```python
from build123d import *

# Parameters (mm, degrees)
BOSS_EXTRUDE1_DEPTH = 22.225
BOSS_EXTRUDE2_DEPTH = 3.175
SKETCH4_R           = 1.000000032
CUT_EXTRUDE2_DEPTH  = 67.374967797
SKETCH5_R           = 2.000000064
CUT_EXTRUDE3_DEPTH  = 69.585879378
SKETCH6_W           = 19.999999878
SKETCH6_H           = 40.899999988
CUT_EXTRUDE4_DEPTH  = 69.585879378
SKETCH7_W           = 1.500000048
SKETCH7_H           = 1.000000032
CUT_EXTRUDE5_DEPTH  = 6.604
CUT_EXTRUDE6_START  = 40.9
SKETCH7_2_W         = 1.500000048
SKETCH7_2_H         = 1.000000032
CUT_EXTRUDE6_DEPTH  = 6.604


with BuildPart() as part:
    # Sketch1 → Boss-Extrude1 (new, symmetric)
    with BuildSketch(Plane.XY):
        Polygon((0, 0), (0, 63.5), (3.175, 63.5), (3.175, 3.175), (16.51, 3.175), (16.51, 0), align=None)
    extrude(amount=BOSS_EXTRUDE1_DEPTH, both=True)

    # Sketch3 → Boss-Extrude2 (add)
    with BuildSketch(Plane.XY.offset(22.225)):
        Polygon((3.175, 63.5), (16.51, 3.175), (3.175, 3.175), align=None)
    boss_extrude2 = extrude(amount=-BOSS_EXTRUDE2_DEPTH)

    # Mirror1: Boss-Extrude2 across plane
    add(boss_extrude2.mirror(Plane.XY))

    # Sketch4 → Cut-Extrude2 (cut, through all)
    with BuildSketch(Plane(origin=(0, 3.175, 0), x_dir=(1, 0, 0), z_dir=(0, 1, 0))):
        with Locations(Location((8.679999912, 12.7, 0), (0, 0, 180))):
            Circle(SKETCH4_R)
        with Locations((8.679999912, -12.7)):
            Circle(SKETCH4_R)
    extrude(amount=-CUT_EXTRUDE2_DEPTH, mode=Mode.SUBTRACT)

    # Sketch5 → Cut-Extrude3 (cut, through all)
    with BuildSketch(Plane(origin=(3.175, 0, 0), x_dir=(0, 0, -1), z_dir=(1, 0, 0))):
        with Locations(Location((-4.953, 5.874999934, 0), (0, 0, 90))):
            Circle(SKETCH5_R)
        with Locations(Location((5.047000066, 5.874999934, 0), (0, 0, 90))):
            Circle(SKETCH5_R)
        with Locations(Location((-4.953, 54.475000016, 0), (0, 0, 90))):
            Circle(SKETCH5_R)
        with Locations(Location((5.047000066, 54.475000016, 0), (0, 0, 90))):
            Circle(SKETCH5_R)
    extrude(amount=-CUT_EXTRUDE3_DEPTH, mode=Mode.SUBTRACT)

    # Sketch6 → Cut-Extrude4 (cut, through all)
    with BuildSketch(Plane(origin=(3.175, 0, 0), x_dir=(0, 0, -1), z_dir=(1, 0, 0))):
        with Locations((0.047000033, 30.174999975)):
            Rectangle(SKETCH6_W, SKETCH6_H)
    extrude(amount=-CUT_EXTRUDE4_DEPTH, mode=Mode.SUBTRACT)

    # Sketch7 → Cut-Extrude5 (cut)
    with BuildSketch(Plane.XZ.offset(-50.624999969)):
        with Locations((2.424999976, 0)):
            Rectangle(SKETCH7_W, SKETCH7_H)
    extrude(amount=-CUT_EXTRUDE5_DEPTH, mode=Mode.SUBTRACT)

    # Sketch7<2> → Cut-Extrude6 (cut)
    with BuildSketch(Plane.XZ.offset(-50.624999969).offset(CUT_EXTRUDE6_START)):
        with Locations((2.424999976, 0)):
            Rectangle(SKETCH7_2_W, SKETCH7_2_H)
    extrude(amount=CUT_EXTRUDE6_DEPTH, mode=Mode.SUBTRACT)


solid = part.part
```
Source: CAD feature listing. Evaluate the final solid. Frame: model axes, mm. A direction names the side the tool comes from. Round coordinates to 2 decimals unless told otherwise and drop trailing zeros. Loops run counter-clockwise (first coordinate to the right, second up) from the corner with the lowest first, then second, coordinate; pieces in that order, holes last.
(1) Material intervals for probe 1 along Z at (x, y) = (8.68, 1.1) (3 decimals); probe 2 along Y at (x, z) = (2.75, 6.5) (3 decimals); probe 3 along Z at (x, y) = (2.75, 33) (3 decimals), sorted ascending.
From the geometry:
probe 1: z = -22.225 to -13.7, -11.7 to 11.7, 13.7 to 22.225
probe 2: y = 0 to 4.607, 7.143 to 9.725, 50.625 to 53.207, 55.743 to 63.5
probe 3: z = -22.225 to -10.047, 9.953 to 22.225
(2) Access query for faces 1 (the flat face through (1, 9.725, 0)), 2 (the flat face through (2, 54, 0.5)), 3 (the flat face through (7, 20, 19.05)). Directions: +Z, -Z, +X, -X, +Y, -Y. A direction counts if a zero-diameter tool reaches every point of the face in a straight line with its end or side. Return the directions, or none.
From the geometry:
face 1: +X, -X
face 2: +X
face 3: +X, +Y
(3) Section query C-C (x = 8.68). Output: boundary loops of the cut face in (y, z) (3 decimals), and give its area (3 significant figures).
From the geometry:
outline: (0, -22.225) - (38.596, -22.225) - (38.596, -19.05) - (3.175, -19.05) - (3.175, -13.7) - (0, -13.7) - close; (0, -11.7) - (3.175, -11.7) - (3.175, 11.7) - (0, 11.7) - close; (0, 13.7) - (3.175, 13.7) - (3.175, 19.05) - (38.596, 19.05) - (38.596, 22.225) - (0, 22.225) - close
area: 353 mm2
(4) Section query D-D (y = 54). Output: boundary loops of the cut face in (x, z) (3 decimals), and give its area (3 significant figures).
From the geometry:
outline: (0, -22.225) - (5.275, -22.225) - (5.275, -19.05) - (3.175, -19.05) - (3.175, -6.99) - (0, -6.99) - close; (0, -3.104) - (3.175, -3.104) - (3.175, -0.5) - (1.675, -0.5) - (1.675, 0.5) - (3.175, 0.5) - (3.175, 3.01) - (0, 3.01) - close; (0, 6.896) - (3.175, 6.896) - (3.175, 19.05) - (5.275, 19.05) - (5.275, 22.225) - (0, 22.225) - close
area: 128 mm2
(5) Pull-direction query (Z, two-part tool) for faces 4 (the flat face through (2, 63.5, 0)), 5 (the cylindrical face through (9.68, 1.61, -12.66)), 6 (the cylindrical face through (1.61, 52.477, -4.959)), 7 (the flat face through (7, 25, 22.225)); classes: +Z half, -Z half, draft (parallel to the pull), parting line (faces both ways), or undercut.
From the geometry:
face 4: draft
face 5: undercut
face 6: undercut
face 7: +Z half
(6) Section query B-B (y = 16). Output: boundary loops of the cut face in (x, z) (3 decimals).
From the geometry:
outline: (0, -22.225) - (13.675, -22.225) - (13.675, -19.05) - (3.175, -19.05) - (3.175, -10.047) - (0, -10.047) - close; (0, 9.953) - (3.175, 9.953) - (3.175, 19.05) - (13.675, 19.05) - (13.675, 22.225) - (0, 22.225) - close
(7) Contact query for flat-ended pins moving along their axis: pin 1 Ø0.5 at (x, z) = (2.5, 0) entering from -Y; pin 2 Ø2.5 at (x, z) = (8.68, 12.7) entering from +Y (3 decimals). Output: stop coordinate, or through.
From the geometry:
pin 1: stops at y = 0
pin 2: stops at y = 3.175
(8) Section query A-A (z = 12.7). Output: boundary loops of the cut face in (x, y) (3 decimals).
From the geometry:
outline: (0, 0) - (7.68, 0) - (7.68, 3.175) - (3.175, 3.175) - (3.175, 63.5) - (0, 63.5) - close; (9.68, 0) - (16.51, 0) - (16.51, 3.175) - (9.68, 3.175) - close
